Input: part model. Units: mm. Frame: model coordinates. A direction names the side the tool comes from. Coordinates: 2 decimals unless noted, no trailing zeros. Order: outer loops, then holes, each group sorted by start corner. A loop starts at its lowest first (then second) coordinate and runs counter-clockwise, first axis right, second up.
from build123d import *

# Parameters (mm, degrees)
F0_W     = 101.7517447472
F0_H     = 95.5048203468
F1_DEPTH = 25
F2_T     = 10
F3_R     = 25.591656965
F4_DEPTH = 25.4
F5_R     = 5.08


# Not quite as in the source:
# - a pattern or mirror of a feature is missing from the dataset's text; its kind, count and spacing are read off the source's solid


with BuildPart() as f1:
    # F0 (on Front) → F1 (new body, symmetric)
    with BuildSketch(Plane.XZ):
        Rectangle(F0_W, F0_H)
    extrude(amount=F1_DEPTH, both=True)

    # F2
    f2_openings = [f1.faces().sort_by_distance(p)[0] for p in [
        (0, 0, 47.75241),
    ]]
    offset(amount=F2_T, openings=f2_openings, kind=Kind.INTERSECTION)

    # F3 (on face) → F4 (join)
    with BuildSketch(Plane.XZ.offset(35)):
        Circle(F3_R)
    f4 = extrude(amount=F4_DEPTH)

    # F4_copies: F4 across plane
    add(f4.mirror(Plane.ZX))

    # F5
    f5_edges = [f1.edges().sort_by_distance(p)[0] for p in [
        (60.875872, 0, 47.75241),
        (0, 35, 47.75241),
        (-60.875872, 0, 47.75241),
        (0, -35, 47.75241),
    ]]
    fillet(f5_edges, radius=F5_R)


solid = f1.part
Item 1: Cut plane D-D on z = -28. Return loops of the section in (x, y).
Response values:
outline: (-60.88, -35) - (60.88, -35) - (60.88, 35) - (-60.88, 35) - close; hole (-50.88, -25) - (50.88, -25) - (50.88, 25) - (-50.88, 25) - close
Item 2: Pin query (flat end, axial travel): pin 1 Ø15 at (x, y) = (-5.5, -7) entering from +Z; pin 2 Ø3 at (x, z) = (16.5, -26.5) entering from +Y; pin 3 Ø10 at (x, y) = (6.5, -48) entering from -Z. Return the tip coordinate at first contact, or that it passes through.
Response values:
pin 1: stops at z = -47.75
pin 2: stops at y = 35
pin 3: stops at z = -25.55
Item 3: Access query for faces 1 (the face through (-18.86, -47.52, 17.3)), 2 (the face through (0, -60.4, 0)), 3 (the face through (-18.86, 47.52, 17.3)), 4 (the face through (50.876, 0, -1)), 5 (the face through (-0.852, 33.472, 46.304)). Directions: +Z, -Z, +X, -X, +Y, -Y. A direction counts if a zero-diameter tool reaches every point of the face in a straight line with its end or side. Return the directions, or none.
Response values:
face 1: -Y
face 2: +Z, -Z, +X, -X, -Y
face 3: +Y
face 4: +Z
face 5: +Z, +X, -X, +Y
Item 4: Cut plane C-C on y = 1.5. Return loops of the section in (x, z).
Response values:
outline: (-60.88, -57.75) - (60.88, -57.75) - (60.88, 42.67) arc R5.08 ccw to (55.8, 47.75) - (50.88, 47.75) - (50.88, -47.75) - (-50.88, -47.75) - (-50.88, 47.75) - (-55.8, 47.75) arc R5.08 ccw to (-60.88, 42.67) - close
Item 5: Ray query, probe 1 along X at (y, z) = (22.5, -40); probe 2 along Y at (x, z) = (-36.5, 32); probe 3 along Y at (x, z) = (8, 23). Return the intervals inside material, ascending.
Response values:
probe 1: x = -60.88 to -50.88, 50.88 to 60.88
probe 2: y = -35 to -25, 25 to 35
probe 3: y = -60.4 to -25, 25 to 60.4
Item 6: Cut plane A-A on z = 0. Return loops of the section in (x, y), then the cut area to 3 significant figures.
Response values:
outline: (-60.88, -35) - (-25.59, -35) - (-25.59, -60.4) - (25.59, -60.4) - (25.59, -35) - (60.88, -35) - (60.88, 35) - (25.59, 35) - (25.59, 60.4) - (-25.59, 60.4) - (-25.59, 35) - (-60.88, 35) - close; hole (-50.88, -25) - (50.88, -25) - (50.88, 25) - (-50.88, 25) - close
area: 6,040 mm2
Item 7: Draft query along X for faces 6 (the face through (-1, 25, 1)), 7 (the face through (-59.35, -0.49, 46.3)), 8 (the face through (0, 60.4, 0)). Return one class per face: pulls with the +X half, pulls with the -X half, needs draft (parallel to the pull), parting line crosses it, or undercut.
Response values:
face 6: undercut
face 7: pulls with the -X half
face 8: needs draft
Item 8: Cut plane B-B on x = 0. Return loops of the section in (y, z).
Response values:
outline: (-60.4, -25.59) - (-35, -25.59) - (-35, -57.75) - (35, -57.75) - (35, -25.59) - (60.4, -25.59) - (60.4, 25.59) - (35, 25.59) - (35, 42.67) arc R5.08 ccw to (29.92, 47.75) - (25, 47.75) - (25, -47.75) - (-25, -47.75) - (-25, 47.75) - (-29.92, 47.75) arc R5.08 ccw to (-35, 42.67) - (-35, 25.59) - (-60.4, 25.59) - close
